from build123d import *

# Parameters (mm, degrees)
CIRCLE_R              = 1.944096
EXTRUDE010_DEPTH      = 100
EXTRUDE008_DEPTH      = 10
EXTRUDE008_DEPTH_BACK = 20


with BuildPart() as extrude010:
    # Circle → Extrude010 (new body)
    with BuildSketch(Plane(origin=(-34.648671, 4.568851, 0), x_dir=(1, 0, 0), z_dir=(0, 0, 1))):
        Circle(CIRCLE_R)
    extrude(amount=EXTRUDE010_DEPTH)


with BuildPart() as cut:
    # Wire002 → Extrude008 (new body, two sides)
    with BuildSketch(Plane(origin=(-41.728547, 12.01263, 0), x_dir=(1, 0, 0), z_dir=(0, 0, 1))) as extrude008_sk:
        Polygon((0, 0), (14.236612, -4.528044), (-0.775791, -10.787191), align=None)
    extrude(amount=EXTRUDE008_DEPTH)
    extrude(extrude008_sk.sketch, amount=-EXTRUDE008_DEPTH_BACK)

    # Cut: cut Extrude010
    add(extrude010.part, mode=Mode.SUBTRACT)


solid = cut.part
Here's how the part is built. I have some questions about the finished solid (model axes, mm). Round coordinates to 2 decimals unless told otherwise and drop trailing zeros. Write each loop counter-clockwise with the first axis right and the second up, starting at its lowest first coordinate (ties: lowest second). Pieces come first, ordered by that corner, then holes. Notation, with made-up numbers: (24, 75.25) -> (41, 75.25) arc R18 ccw to (41, 83.25) -> close; hole circle Ø3 at (3, 60). An arc over 180 degrees is marked (long way). One line per item, written item: value.
1) Suppose I cut it at D-D on x = -29.75. List the corners of the cut face in (y, z) for me.
Filled sheet:
outline: (6.54, -20) -> (8.2, -20) -> (8.2, 10) -> (6.54, 10) -> close
2) We'd pull the mould along X, two halves only. Please class faces 1 (the face through (-35.36, 6.38, 4.93)), 2 (the face through (-38, 7, -20)), 3 (the face through (-42.122, 6.544, -4.79)), 4 (the face through (-35, 5, 0)): released by +X, released by -X, zero draft, split by the parting line, or undercut.
Filled sheet:
face 1: undercut
face 2: zero draft
face 3: released by -X
face 4: undercut
3) Suppose I cut it at C-C on y = 2. List the corners of the cut face in (x, z) for me.
Filled sheet:
outline: (-42.45, -20) -> (-40.65, -20) -> (-40.65, 10) -> (-42.45, 10) -> close
4) I'm going to push flat-ended pins straight in: pin 1 Ø6 at (x, z) = (-36.5, -9.5) entering from -Y; pin 2 Ø4 at (y, z) = (2.5, -7) entering from +X; pin 3 Ø6 at (x, z) = (-37, -6) entering from -Y. Where does each tip first touch, or does it pass through?
Filled sheet:
pin 1: stops at y = 2.48
pin 2: stops at x = -34.65
pin 3: stops at y = 2.27
5) If I drill on line 1 (Z direction, x = -35.75, y = 6); line 2 (Y direction, x = -36.75, z = 1.75); line 3 (Y direction, x = -27.75, z = 8.75), over which ranges is the centre line in solid material (lowest first)? Write a range as [from, to].
Filled sheet:
line 1: z = [-20, 0]
line 2: y = [3.62, 10.43]
line 3: y = [7.38, 7.57]
6) Suppose I cut it at A-A on z = -5.75. List the corners of the cut face in (x, y) for me, plus the area to 3 significant figures.
Filled sheet:
outline: (-42.5, 1.23) -> (-27.49, 7.48) -> (-41.73, 12.01) -> close
area: 78.5 mm2
7) Suppose I cut it at B-B on x = -35.75. List the corners of the cut face in (y, z) for me.
Filled sheet:
outline: (4.04, -20) -> (10.11, -20) -> (10.11, 10) -> (6.17, 10) -> (6.17, 0) -> (4.04, 0) -> close
